Job drawing, mm, ordinate dimensions from the low corner. One solid piece. A direction names the side the tool comes from. Round coordinates to 2 decimals unless told otherwise and drop trailing zeros. Write each loop counter-clockwise with the first axis right and the second up, starting at its lowest first coordinate (ties: lowest second). Pieces come first, ordered by that corner, then holes.
1) Saw through at C-C (y = 54). Write the cut outline in (x, z).
2) Saw through at B-B (x = 74). Write the cut outline in (y, z), plus the area to 3 significant figures.
3) Saw through at D-D (z = 117). Write the cut outline in (x, y), plus the area to 3 significant figures.
4) Flat gauge pins, fed straight in: pin 1 (1.5 mm diameter, centred on y = 94, z = 18, fed in from -X); pin 2 (22 mm diameter, centred on y = 8, z = 27.5, fed in from -X); pin 3 (1.5 mm diameter, centred on y = 23.5, z = 32, fed in from -X) (1 decimal); pin 4 (2 mm diameter, centred on y = 37, z = 122.5, fed in from -X). Where does each tip first touch, or does it go through?
5) Saw through at A-A (z = 23). State how many separate pieces and enclosed holes the cut face has, plus the area to 3 significant figures.
6) Pull direction Y, two halves, no side cores. Call the marked faces 1, 2, 3 and 4: +Y half, -Y half, draft (parallel to the pull), parting line (faces both ways), or undercut.
7) Wall check: probe 1 along Z at (x, y) = (59, 96); probe 2 along Z at (x, y) = (143, 12.5); probe 3 along Y at (x, z) = (56.5, 17.5) (1 decimal). Give the ranges that are in metal, low to high.
8) Which spindle directions (+Z, -Z, +X, -X, +Y, -Y) get a long thin tool onto all of the face, cutting with end or side? Do the marked faces 5, 6 and 7. Say none if no direction does.
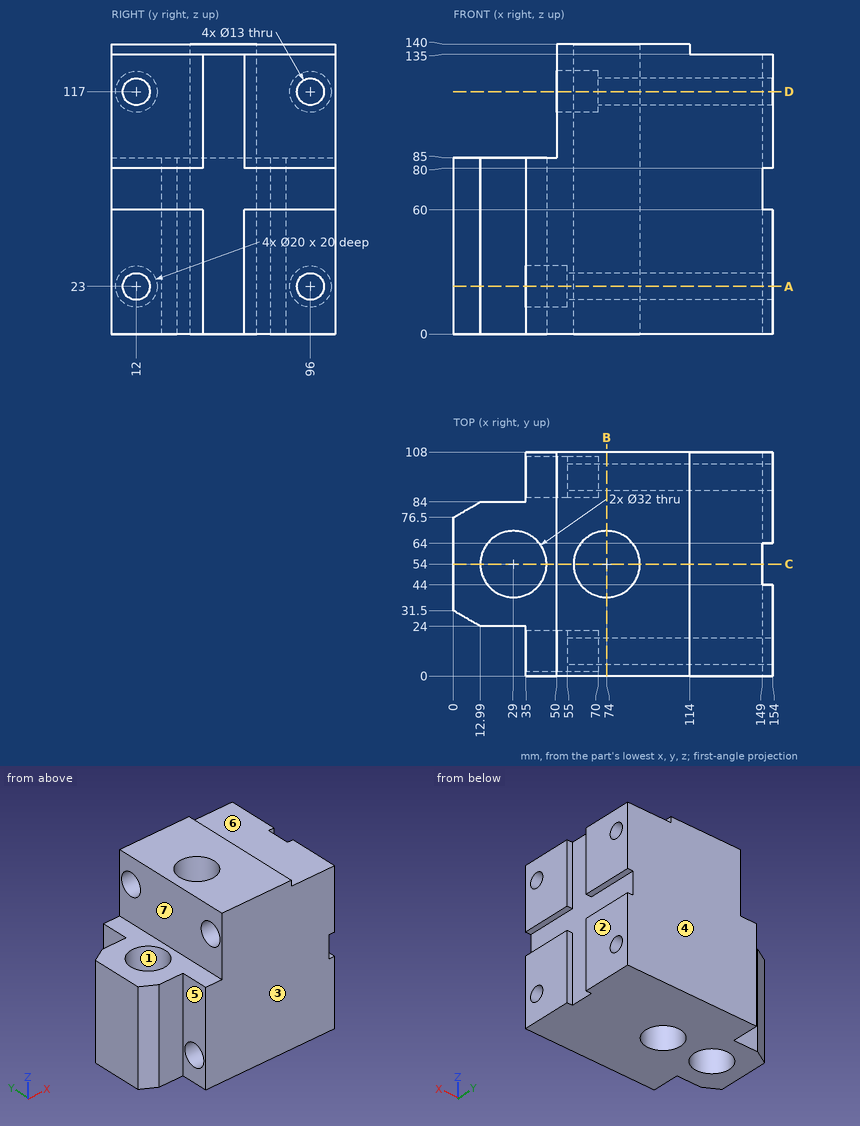
Evaluation:
1. outline: (0, 0) - (13, 0) - (13, 85) - (0, 85) - close; (45, 0) - (58, 0) - (58, 140) - (50, 140) - (50, 85) - (45, 85) - close; (90, 0) - (149, 0) - (149, 135) - (114, 135) - (114, 140) - (90, 140) - close
2. outline: (0, 0) - (38, 0) - (38, 140) - (0, 140) - close; (70, 0) - (108, 0) - (108, 140) - (70, 140) - close; hole circle Ø13 at (12, 23); hole circle Ø13 at (12, 117); hole circle Ø13 at (96, 23); hole circle Ø13 at (96, 117)
2. area: 10,100 mm2
3. outline: (50, 0) - (154, 0) - (154, 5.5) - (70, 5.5) - (70, 2) - (50, 2) - close; (50, 22) - (70, 22) - (70, 18.5) - (154, 18.5) - (154, 44) - (149, 44) - (149, 64) - (154, 64) - (154, 89.5) - (70, 89.5) - (70, 86) - (50, 86) - close; (50, 106) - (70, 106) - (70, 102.5) - (154, 102.5) - (154, 108) - (50, 108) - close; hole circle Ø32 at (74, 54)
3. area: 7,340 mm2
4. pin 1: passes through
4. pin 2: stops at x = 35
4. pin 3: stops at x = 12.6
4. pin 4: stops at x = 50
5. separate pieces: 3
5. enclosed holes: 2
5. area: 9,770 mm2
6. face 1: undercut
6. face 2: draft
6. face 3: -Y half
6. face 4: +Y half
7. probe 1: z = 0 to 16.5, 29.5 to 107, 127 to 140
7. probe 2: z = 0 to 16.52, 29.48 to 110.52, 123.48 to 135
7. probe 3: y = 0 to 8.5, 15.5 to 92.5, 99.5 to 108
8. face 5: +Z, -Z, -X, -Y
8. face 6: +Z, +X, +Y, -Y
8. face 7: +Z, -X, +Y, -Y
